Verification items for the finished model (mm, model axes). A direction names the side the tool comes from. Coordinates: 2 decimals unless noted, no trailing zeros. Write each loop counter-clockwise with the first axis right and the second up, starting at its lowest first coordinate (ties: lowest second). Pieces come first, ordered by that corner, then holes. Notation, with made-up numbers: (20.25, 87.5) - (65.25, 87.5) arc R23 ccw to (65.25, 97.5) - close; hole circle Ø1 at (21, 19.5). An arc over 180 degrees is marked (long way). Answer as CSV lines item,"result". Start each with the question number.
```python
from build123d import *

# Parameters (mm, degrees)
F0_R     = 1
F1_DEPTH = 11
F2_R     = 0.8
F3_DEPTH = 7
F4_SIZE  = 0.1
F5_SIZE2 = 0.133975
F5_SIZE  = 0.5


with BuildPart() as f1:
    # F0 (on Top) → F1 (new body)
    with BuildSketch(Plane.XY):
        Circle(F0_R)
    extrude(amount=F1_DEPTH)

    # F2 (on face) → F3 (join)
    with BuildSketch(Plane.XY.offset(11)):
        Circle(F2_R)
    extrude(amount=F3_DEPTH)

    # F4
    f4_edges = [f1.edges().sort_by_distance(p)[0] for p in [
        (-1, 0, 0),
    ]]
    chamfer(f4_edges, length=F4_SIZE)

    # F5
    f5_edges = [f1.edges().sort_by_distance(p)[0] for p in [
        (-0.8, 0, 18),
    ]]
    chamfer(f5_edges, length=F5_SIZE, length2=F5_SIZE2)


solid = f1.part
```
1. Cross-section at C-C (z = 15.5). Record the cut outline in (x, y), and give its area (3 significant figures).
2. Cross-section at A-A (y = 0). Record the cut outline in (x, z).
3. Access from +Z, -Z, +X, -X, +Y, -Y to the whole of each face (thin tool, end or side, straight path). Record for faces 1 (the face through (0, 0, 0)), 2 (the face through (-0.63, -0.49, 14.2)).
4. Cross-section at D-D (z = 6.25). Record the cut outline in (x, y), and give its area (3 significant figures).
5. Scan lines: line 1 along Z through (x, y) = (0.15, -0.85); line 2 along X through (y, z) = (0.6, 8.5); line 3 along X through (y, z) = (-0.05, 10.25). Record each from-to range of solid material in increasing order. Write a range as from..to.
Completed:
1,outline,"circle Ø1.6 at (0, 0)"
1,area,"2.01 mm2"
2,outline,"(-1, 0.1) - (-0.9, 0) - (0.9, 0) - (1, 0.1) - (1, 11) - (0.8, 11) - (0.8, 17.5) - (0.67, 18) - (-0.67, 18) - (-0.8, 17.5) - (-0.8, 11) - (-1, 11) - close"
3,face 1,"-Z, +X, -X, +Y, -Y"
3,face 2,"+Z"
4,outline,"circle Ø2 at (0, 0)"
4,area,"3.14 mm2"
5,line 1,"z = 0..11"
5,line 2,"x = -0.8..0.8"
5,line 3,"x = -1..1"
